The listing builds one solid part. Answer for the finished solid, in the listing's coordinates (mm). Face numbers are marked on the shaded views. A direction names the side the tool comes from. Coordinates: 2 decimals unless noted, no trailing zeros. Order: outer loops, then holes, each group sorted by start corner. A loop starts at its lowest first (then second) coordinate and runs counter-clockwise, first axis right, second up. Notation, with made-up numbers: (38, 51) -> (50, 51) arc R30 cw to (50, 83) -> close; hole circle Ø2 at (-14, 77.25). An arc over 180 degrees is marked (long way). Return JSON: item names as keys, results as strings.
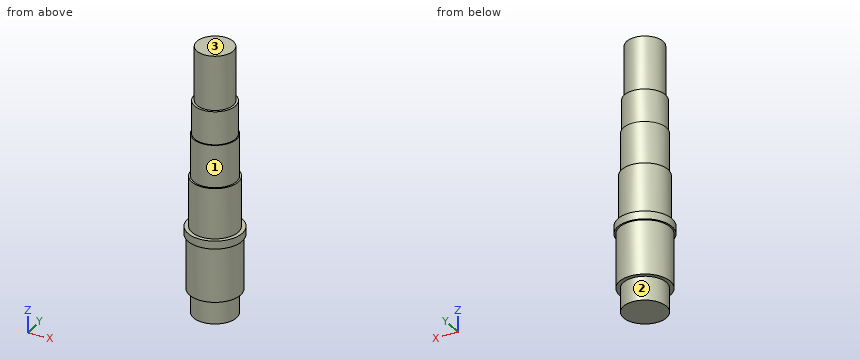
from build123d import *

# Parameters (mm, degrees)
SKETCH_1_R      = 32.5
EXTRUDE_1_DEPTH = 36
SKETCH_2_R      = 38.5
EXTRUDE_2_DEPTH = 82
SKETCH_3_R      = 41
EXTRUDE_3_DEPTH = 12
SKETCH_4_R      = 35
EXTRUDE_4_DEPTH = 76
SKETCH_5_R      = 32.5
EXTRUDE_5_DEPTH = 64
SKETCH_6_R      = 31
EXTRUDE_6_DEPTH = 50
SKETCH_7_R      = 27.5
EXTRUDE_7_DEPTH = 82


with BuildPart() as part:
    # 草图1 → 凸台-拉伸1 (new body)
    with BuildSketch(Plane.XY):
        Circle(SKETCH_1_R)
    extrude(amount=EXTRUDE_1_DEPTH)

    # 草图2 → 凸台-拉伸2 (add)
    with BuildSketch(Plane.XY.offset(36)):
        Circle(SKETCH_2_R)
    extrude(amount=EXTRUDE_2_DEPTH)

    # 草图3 → 凸台-拉伸3 (add)
    with BuildSketch(Plane.XY.offset(118)):
        Circle(SKETCH_3_R)
    extrude(amount=EXTRUDE_3_DEPTH)

    # 草图4 → 凸台-拉伸4 (add)
    with BuildSketch(Plane.XY.offset(130)):
        Circle(SKETCH_4_R)
    extrude(amount=EXTRUDE_4_DEPTH)

    # 草图5 → 凸台-拉伸5 (add)
    with BuildSketch(Plane.XY.offset(206)):
        Circle(SKETCH_5_R)
    extrude(amount=EXTRUDE_5_DEPTH)

    # 草图6 → 凸台-拉伸6 (add)
    with BuildSketch(Plane.XY.offset(270)):
        Circle(SKETCH_6_R)
    extrude(amount=EXTRUDE_6_DEPTH)

    # 草图7 → 凸台-拉伸7 (add)
    with BuildSketch(Plane.XY.offset(320)):
        Circle(SKETCH_7_R)
    extrude(amount=EXTRUDE_7_DEPTH)


solid = part.part
1. The part is cut by section C-C on z = 351. Give the vertices of the cut face in (x, y).
Answer block:
{"outline": "circle Ø55 at (0, 0)"}
2. The part is cut by section A-A on x = 0. Give the vertices of the cut face in (y, z).
Answer block:
{"outline": "(-41, 118) -> (-38.5, 118) -> (-38.5, 36) -> (-32.5, 36) -> (-32.5, 0) -> (32.5, 0) -> (32.5, 36) -> (38.5, 36) -> (38.5, 118) -> (41, 118) -> (41, 130) -> (35, 130) -> (35, 206) -> (32.5, 206) -> (32.5, 270) -> (31, 270) -> (31, 320) -> (27.5, 320) -> (27.5, 402) -> (-27.5, 402) -> (-27.5, 320) -> (-31, 320) -> (-31, 270) -> (-32.5, 270) -> (-32.5, 206) -> (-35, 206) -> (-35, 130) -> (-41, 130) -> close"}
3. For the marked faces 1, 2 and 3, determine the directions among +Z, -Z, +X, -X, +Y, -Y from which every point of the face is accessible in a straight line to the end or side of a thin tool.
Answer block:
{"face 1": "+Z", "face 2": "-Z", "face 3": "+Z, +X, -X, +Y, -Y"}
4. The part is cut by section D-D on z = 134. Give the vertices of the cut face in (x, y), and give its area (3 significant figures).
Answer block:
{"outline": "circle Ø70 at (0, 0)", "area": "3,850 mm2"}
5. Consider line 1 (Z direction, x = -25, y = -19); line 2 (Y direction, x = 0, z = 171.5); line 3 (Z direction, x = 29, y = 5). Determine where each line is inside the solid, lowest interval first. Write a range as from..to.
Answer block:
{"line 1": "z = 0..270", "line 2": "y = -35..35", "line 3": "z = 0..320"}
6. Each of these flat-tipped pins is pushed along its axis until it touches: pin 1 Ø4 at (y, z) = (-6.5, 188.5) entering from -X; pin 2 Ø10 at (y, z) = (14.5, 229) entering from -X; pin 3 Ø5 at (x, z) = (11.5, 234.5) entering from -Y. Where does it stop, or does it pass through?
Answer block:
{"pin 1": "stops at x = -34.71", "pin 2": "stops at x = -31.08", "pin 3": "stops at y = -31.23"}
